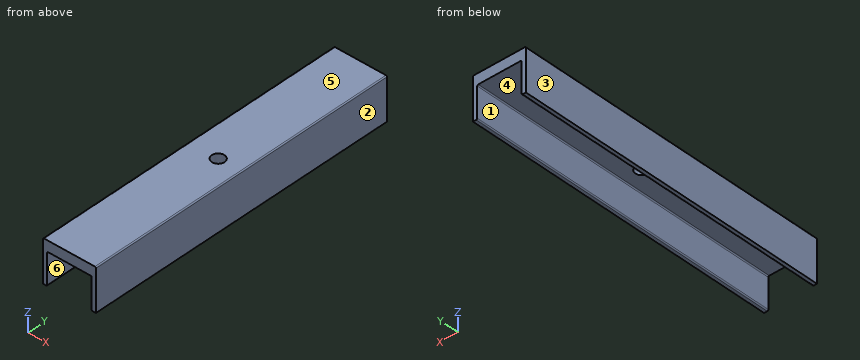
from build123d import *

# Parameters (mm, degrees)
F1_DEPTH = 75
F2_R     = 3
F3_DEPTH = 5
F4_R     = 0.5


with BuildPart() as f1:
    # F0 (on Front) → F1 (new body, symmetric)
    with BuildSketch(Plane.XZ):
        Polygon((25, 20), (0, 20), (0, 0), (2, 0), (2, 15), (23, 15), (23, 0), (25, 0), align=None)
    extrude(amount=F1_DEPTH, both=True)

    # F2 (on face) → F3 (cut, through all)
    with BuildSketch(Plane.XY.offset(20)):
        with Locations((14, 0)):
            Circle(F2_R)
    extrude(amount=-F3_DEPTH, mode=Mode.SUBTRACT)

    # F4
    f4_edges = [f1.edges().sort_by_distance(p)[0] for p in [
        (0, 0, 20),
        (25, 0, 20),
        (2, 0, 0),
        (2, 0, 15),
        (23, 0, 15),
        (23, 0, 0),
    ]]
    fillet(f4_edges, radius=F4_R)


solid = f1.part
CAD build for the part. Positions are in the model's coordinates, mm. Face numbers are marked on the shaded views. A direction names the side the tool comes from. Coordinates: 2 decimals unless noted, no trailing zeros. Order: outer loops, then holes, each group sorted by start corner. A loop starts at its lowest first (then second) coordinate and runs counter-clockwise, first axis right, second up.
Item 1: Band-saw the part on B-B on z = 4.25. List the corners of the cut face in (x, y), plus the area to 3 significant figures.
Check sheet entries:
outline: (0, -75) - (2, -75) - (2, 75) - (0, 75) - close; (23, -75) - (25, -75) - (25, 75) - (23, 75) - close
area: 600 mm2
Item 2: Drill centre lines: L1, parallel to X at y = 50, z = 14.5; L2, parallel to Y at x = 14, z = 17.2; L3, parallel to Z at x = 5, y = 59. Where is each one in solid material? Low to high.
Check sheet entries:
L1: x = 0 to 2, 23 to 25
L2: y = -75 to -3, 3 to 75
L3: z = 15 to 20
Item 3: Band-saw the part on C-C on x = 14. List the corners of the cut face in (y, z), plus the area to 3 significant figures.
Check sheet entries:
outline: (-75, 15) - (-3, 15) - (-3, 20) - (-75, 20) - close; (3, 15) - (75, 15) - (75, 20) - (3, 20) - close
area: 720 mm2
Item 4: Band-saw the part on D-D on y = -39.5. List the corners of the cut face in (x, z), plus the area to 3 significant figures.
Check sheet entries:
outline: (0, 0) - (1.5, 0) arc R0.5 ccw to (2, 0.5) - (2, 14.5) arc R0.5 cw to (2.5, 15) - (22.5, 15) arc R0.5 cw to (23, 14.5) - (23, 0.5) arc R0.5 ccw to (23.5, 0) - (25, 0) - (25, 19.5) arc R0.5 ccw to (24.5, 20) - (0.5, 20) arc R0.5 ccw to (0, 19.5) - close
area: 185 mm2
Item 5: Pin check, flat tip, straight feed: pin 1 Ø7 at (x, y) = (14, 0) entering from -Z. Stop position of the tip, or through.
Check sheet entries:
pin 1: stops at z = 15
Item 6: Two-plate mould, pull along X, no slides. Class the marked faces 3, 4, 5 and 6: +X half, -X half, draft (parallel to the pull), parting line (faces both ways), or undercut.
Check sheet entries:
face 3: -X half
face 4: undercut
face 5: draft
face 6: undercut
Item 7: 3-axis set-ups, long thin cutter, end or side, ignore diameter. For the marked faces 1 and 2: which of +Z, -Z, +X, -X, +Y, -Y reach the whole face in a straight line?
Check sheet entries:
face 1: -Z, +Y, -Y
face 2: +Z, -Z, +X, +Y, -Y
Item 8: Band-saw the part on A-A on y = 0. List the corners of the cut face in (x, z), plus the area to 3 significant figures.
Check sheet entries:
outline: (0, 0) - (1.5, 0) arc R0.5 ccw to (2, 0.5) - (2, 14.5) arc R0.5 cw to (2.5, 15) - (11, 15) - (11, 20) - (0.5, 20) arc R0.5 ccw to (0, 19.5) - close; (17, 15) - (22.5, 15) arc R0.5 cw to (23, 14.5) - (23, 0.5) arc R0.5 ccw to (23.5, 0) - (25, 0) - (25, 19.5) arc R0.5 ccw to (24.5, 20) - (17, 20) - close
area: 155 mm2
